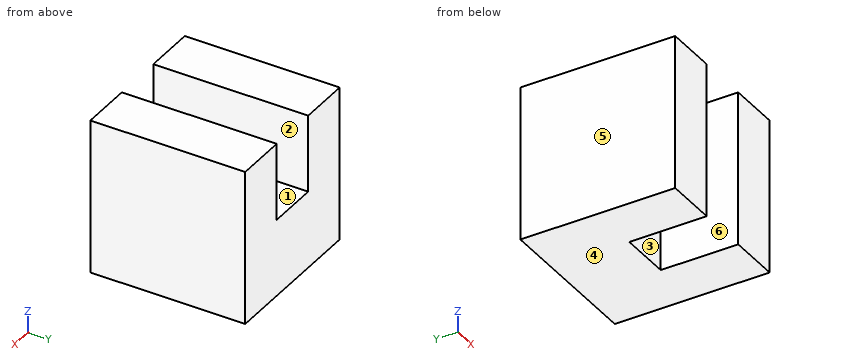
```python
from build123d import *

# Parameters (mm, degrees)
F0_W     = 76.2
F0_H     = 76.2
F1_DEPTH = 25.4
F2_W     = 38.1
F2_H     = 38.1
F3_DEPTH = 25.4
F4_W     = 76.2
F4_H     = 76.2
F5_DEPTH = 25.4


with BuildPart() as f1:
    # F0 (on Right) → F1 (new body)
    with BuildSketch(Plane.YZ):
        Rectangle(F0_W, F0_H)
    extrude(amount=F1_DEPTH)

    # F2 (on face) → F3 (join)
    with BuildSketch(Plane.YZ.offset(25.4)):
        with Locations((19.05, -19.05)):
            Rectangle(F2_W, F2_H)
    extrude(amount=F3_DEPTH)

    # F4 (on face) → F5 (join)
    with BuildSketch(Plane.YZ.offset(50.8)):
        Rectangle(F4_W, F4_H)
    extrude(amount=F5_DEPTH)


solid = f1.part
```
Here's how the part is built. I have some questions about the finished solid (model axes, mm). Face numbers are marked on the shaded views. A direction names the side the tool comes from. Give positions to 0.01 mm unless a question says otherwise; leave off trailing zeros. Write each loop counter-clockwise with the first axis right and the second up, starting at its lowest first coordinate (ties: lowest second). Pieces come first, ordered by that corner, then holes. Notation, with made-up numbers: (33, -21) -> (66, -21) arc R20 ccw to (66, -15) -> close; hole circle Ø8 at (49.5, 44.5). An arc over 180 degrees is marked (long way). Write each question's results on one line, items separated by ' | '.
Item 1: Suppose I cut it at A-A on z = 28. Write out the boundary of the cut face in (x, y).
Output:
outline: (0, -38.1) -> (25.4, -38.1) -> (25.4, 38.1) -> (0, 38.1) -> close; (50.8, -38.1) -> (76.2, -38.1) -> (76.2, 38.1) -> (50.8, 38.1) -> close
Item 2: If I drill on L1, parallel to X at y = -31, z = 24; L2, parallel to Z at x = 43, y = 12.5; L3, parallel to Y at x = 32, z = -19.5, over which ranges is the centre line in solid material (lowest first)?
Output:
L1: x = 0 to 25.4, 50.8 to 76.2 | L2: z = -38.1 to 0 | L3: y = 0 to 38.1
Item 3: On a 3-axis mill with a long thin cutter (end or side, diameter ignored), from which of +Z, -Z, +X, -X, +Y, -Y can I reach the whole of each face in a straight line? I mean the marked faces 1, 2 and 3. Say none if no direction works.
Output:
face 1: +Z, +Y, -Y | face 2: +Z, -Y | face 3: +Z, -Z, -Y
Item 4: For pin 1 Ø12.5 at (x, y) = (34.5, 18) entering from +Z; pin 2 Ø12.5 at (x, z) = (35, -27) entering from -Y, each with a flat end and sliding along its axis, tell me the tip position at first contact or that it passes through.
Output:
pin 1: stops at z = 0 | pin 2: stops at y = 0
Item 5: Suppose I cut it at D-D on z = -13.5. Write out the boundary of the cut face in (x, y), plus the area to 3 significant figures.
Output:
outline: (0, -38.1) -> (25.4, -38.1) -> (25.4, 0) -> (50.8, 0) -> (50.8, -38.1) -> (76.2, -38.1) -> (76.2, 38.1) -> (0, 38.1) -> close | area: 4,840 mm^2
Item 6: We'd pull the mould along X, two halves only. Please class the marked faces 4, 5 and 6: pulls with the +X half, pulls with the -X half, needs draft (parallel to the pull), parting line crosses it, or undercut.
Output:
face 4: needs draft | face 5: pulls with the -X half | face 6: undercut
Item 7: Suppose I cut it at C-C on y = 10. Write out the boundary of the cut face in (x, z), plus the area to 3 significant figures.
Output:
outline: (0, -38.1) -> (76.2, -38.1) -> (76.2, 38.1) -> (50.8, 38.1) -> (50.8, 0) -> (25.4, 0) -> (25.4, 38.1) -> (0, 38.1) -> close | area: 4,840 mm^2
